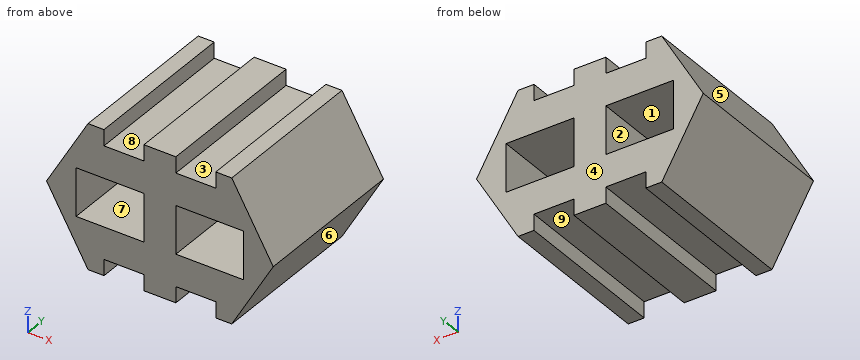
from build123d import *

# Parameters (mm, degrees)
F0_W     = 53.975
F0_H     = 38.1
F1_DEPTH = 127


with BuildPart() as f1:
    # F0 (on Front) → F1 (new body)
    with BuildSketch(Plane.XZ):
        Polygon((12.7, 0), (0, 0), (-32.995568, -57.15), (0, -114.3), (12.7, -114.3), (12.7, -101.6), (44.45, -101.6), (44.45, -114.3), (69.85, -114.3), (69.85, -101.6), (101.6, -101.6), (101.6, -114.3), (114.3, -114.3), (147.295568, -57.15), (114.3, 0), (101.6, 0), (101.6, -12.7), (69.85, -12.7), (69.85, 0), (44.45, 0), (44.45, -12.7), (12.7, -12.7), align=None)
        with Locations((17.4625, -57.15)):
            Rectangle(F0_W, F0_H, mode=Mode.SUBTRACT)
        with Locations((96.8375, -57.15)):
            Rectangle(F0_W, F0_H, mode=Mode.SUBTRACT)
    extrude(amount=F1_DEPTH)


solid = f1.part
Input: part model. Units: mm. Frame: model coordinates. Face numbers are marked on the shaded views. A direction names the side the tool comes from. Give positions to 0.01 mm unless a question says otherwise; leave off trailing zeros. Order: outer loops, then holes, each group sorted by start corner. A loop starts at its lowest first (then second) coordinate and runs counter-clockwise, first axis right, second up. Notation, with made-up numbers: M 5,31 L 46,31 A28 ccw 46,65 Z; hole C 56.25,-32 d10. An arc over 180 degrees is marked long. Answer as a JSON object with one key per item and string values.
1. Cut plane A-A, the plane x = 10. Output: boundary loops of the cut face in (y, z), and give its area (3 significant figures).
Result sheet:
{"outline": "M -127,-114.3 L 0,-114.3 L 0,-76.2 L -127,-76.2 Z; M -127,-38.1 L 0,-38.1 L 0,0 L -127,0 Z", "area": "9,680 mm²"}
2. Reachability of the marked faces 5, 6, 7, 8 and 9 from +Z, -Z, +X, -X, +Y, -Y: full face, straight path, thin tool, end or side. Return the list, or none.
Result sheet:
{"face 5": "+Z, -X, +Y, -Y", "face 6": "-Z, +X, +Y, -Y", "face 7": "+Y, -Y", "face 8": "+Z, +Y, -Y", "face 9": "-Z, +Y, -Y"}
3. Cut plane D-D, the plane z = -59.5. Output: boundary loops of the cut face in (x, y) (3 decimals), and give its area (3 significant figures).
Result sheet:
{"outline": "M -31.639,-127 L -9.525,-127 L -9.525,0 L -31.639,0 Z; M 44.45,-127 L 69.85,-127 L 69.85,0 L 44.45,0 Z; M 123.825,-127 L 145.939,-127 L 145.939,0 L 123.825,0 Z", "area": "8,840 mm²"}
4. First-contact query: P1, Ø5, axis at y = -80, z = -79.5, coming from the +X side; P2, Ø14, axis at y = -62.5, z = -105, coming from the -X side; P3, Ø10, axis at y = -56.5, z = -107, coming from the +X side. Flat tips, straight axial feed; report the tip coordinate or a pass-through.
Result sheet:
{"P1": "x = 135.84", "P2": "x = -9.41", "P3": "x = 121.4"}
5. Cut plane B-B, the plane z = -9.5. Output: boundary loops of the cut face in (x, y).
Result sheet:
{"outline": "M -5.48,-127 L 12.7,-127 L 12.7,0 L -5.48,0 Z; M 44.45,-127 L 69.85,-127 L 69.85,0 L 44.45,0 Z; M 101.6,-127 L 119.78,-127 L 119.78,0 L 101.6,0 Z"}
6. Pull-direction query (Z, two-part tool) for the marked faces 1, 2, 3 and 4; classes: +Z half, -Z half, draft (parallel to the pull), parting line (faces both ways), or undercut.
Result sheet:
{"face 1": "undercut", "face 2": "undercut", "face 3": "+Z half", "face 4": "draft"}
7. Ray query, line 1 (Z direction, x = 79, y = -51); line 2 (X direction, y = -104.5, z = -6); line 3 (X direction, y = -35, z = -62) (3 decimals). Return the intervals inside material, ascending. Write a range as [from, to].
Result sheet:
{"line 1": "[-101.6, -76.2], [-38.1, -12.7]", "line 2": "[-3.46, 12.7], [44.45, 69.85], [101.6, 117.76]", "line 3": "[-30.195, -9.525], [44.45, 69.85], [123.825, 144.495]"}
8. Cut plane C-C, the plane y = -89. State how many separate pieces and enclosed holes the cut face has, and give its area (3 significant figures).
Result sheet:
{"separate pieces": "1", "enclosed holes": "2", "area": "11,100 mm²"}
